Could you check a few things on this model? Use its own coordinates, in mm. Face numbers are marked on the shaded views. A direction names the side the tool comes from. Give positions to 0.01 mm unless a question says otherwise; leave off trailing zeros. Write each loop counter-clockwise with the first axis right and the second up, starting at its lowest first coordinate (ties: lowest second). Pieces come first, ordered by that corner, then holes. Notation, with made-up numbers: M -1.5,-16.5 L 51.5,-16.5 A21 ccw 51.5,13.5 Z; hole C -36.5,56 d7. An arc over 180 degrees is marked long. One line per item, written item: value.
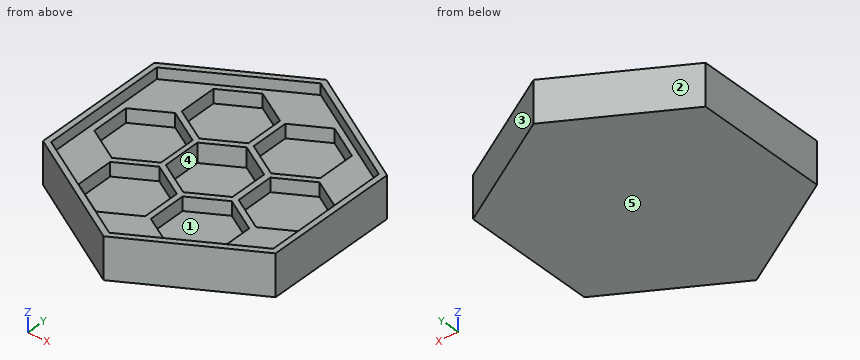
```python
from build123d import *

# Parameters (mm, degrees)
F1_DEPTH = 15
F2_DEPTH = 11
F3_DEPTH = 4
F4_DEPTH = 2


with BuildPart() as f1:
    # F0 (on Top) → F1 (new body)
    with BuildSketch(Plane.XY):
        Polygon((42.0776976909, 24.1136342559), (0.1558290023, 48.4971722611), (-41.9218686887, 24.3835380051), (-42.0776976909, -24.1136342559), (-0.1558290023, -48.4971722611), (41.9218686887, -24.3835380051), align=None)
        Polygon((-40, 23.0940107676), (0, 46.1880215352), (40, 23.0940107676), (40, -23.0940107676), (0, -46.1880215352), (-40, -23.0940107676), align=None, mode=Mode.SUBTRACT)
    extrude(amount=F1_DEPTH)

    # F0 (on Top) → F2 (join)
    with BuildSketch(Plane.XY):
        Polygon((40, 23.0940107676), (0, 46.1880215352), (-40, 23.0940107676), (-40, -23.0940107676), (0, -46.1880215352), (40, -23.0940107676), align=None)
        Polygon((-12.8555934585, -8.7122082831), (-0.8555934585, -15.6404115134), (-0.8555934585, -29.4968179739), (-12.8555934585, -36.4250212042), (-24.8555934585, -29.4968179739), (-24.8555934585, -15.6404115134), align=None, mode=Mode.SUBTRACT)
        Polygon((13.1444065415, -8.6082997926), (25.1444065415, -15.5365030229), (25.1444065415, -29.3929094834), (13.1444065415, -36.3211127137), (1.1444065415, -29.3929094834), (1.1444065415, -15.5365030229), align=None, mode=Mode.SUBTRACT)
        Polygon((-25.7656060661, 13.8564064606), (-13.7656060661, 6.9282032303), (-13.7656060661, -6.9282032303), (-25.7656060661, -13.8564064606), (-37.7656060661, -6.9282032303), (-37.7656060661, 6.9282032303), align=None, mode=Mode.SUBTRACT)
        Polygon((-12.882803033, 36.4407306594), (-0.882803033, 29.5125274291), (-0.882803033, 15.6561209685), (-12.882803033, 8.7279177383), (-24.882803033, 15.6561209685), (-24.882803033, 29.5125274291), align=None, mode=Mode.SUBTRACT)
        Polygon((0, 13.8564064606), (12, 6.9282032303), (12, -6.9282032303), (0, -13.8564064606), (-12, -6.9282032303), (-12, 6.9282032303), align=None, mode=Mode.SUBTRACT)
        Polygon((13.117196967, 36.3054032585), (25.117196967, 29.3772000282), (25.117196967, 15.5207935677), (13.117196967, 8.5925903374), (1.117196967, 15.5207935677), (1.117196967, 29.3772000282), align=None, mode=Mode.SUBTRACT)
        Polygon((26.2343939339, 13.8564064606), (38.2343939339, 6.9282032303), (38.2343939339, -6.9282032303), (26.2343939339, -13.8564064606), (14.2343939339, -6.9282032303), (14.2343939339, 6.9282032303), align=None, mode=Mode.SUBTRACT)
    extrude(amount=F2_DEPTH)

    # F0 (on Top) → F3 (join)
    with BuildSketch(Plane.XY):
        Polygon((25.117196967, 15.5207935677), (25.117196967, 29.3772000282), (13.117196967, 36.3054032585), (1.117196967, 29.3772000282), (1.117196967, 15.5207935677), (13.117196967, 8.5925903374), align=None)
        Polygon((-0.882803033, 15.6561209685), (-0.882803033, 29.5125274291), (-12.882803033, 36.4407306594), (-24.882803033, 29.5125274291), (-24.882803033, 15.6561209685), (-12.882803033, 8.7279177383), align=None)
        Polygon((-13.7656060661, -6.9282032303), (-13.7656060661, 6.9282032303), (-25.7656060661, 13.8564064606), (-37.7656060661, 6.9282032303), (-37.7656060661, -6.9282032303), (-25.7656060661, -13.8564064606), align=None)
        Polygon((12, -6.9282032303), (12, 6.9282032303), (0, 13.8564064606), (-12, 6.9282032303), (-12, -6.9282032303), (0, -13.8564064606), align=None)
        Polygon((38.2343939339, -6.9282032303), (38.2343939339, 6.9282032303), (26.2343939339, 13.8564064606), (14.2343939339, 6.9282032303), (14.2343939339, -6.9282032303), (26.2343939339, -13.8564064606), align=None)
        Polygon((25.1444065415, -29.3929094834), (25.1444065415, -15.5365030229), (13.1444065415, -8.6082997926), (1.1444065415, -15.5365030229), (1.1444065415, -29.3929094834), (13.1444065415, -36.3211127137), align=None)
        Polygon((-0.8555934585, -29.4968179739), (-0.8555934585, -15.6404115134), (-12.8555934585, -8.7122082831), (-24.8555934585, -15.6404115134), (-24.8555934585, -29.4968179739), (-12.8555934585, -36.4250212042), align=None)
    extrude(amount=F3_DEPTH)

    # F4 (add): faces of the model
    f4_faces = [f1.faces().sort_by_distance(p)[0] for p in [
        (-25.7656060661, 0, 4),
        (-12.882803033, 22.5843241988, 4),
        (13.117196967, 22.448996798, 4),
        (26.2343939339, 0, 4),
        (13.1444065415, -22.4647062531, 4),
        (-12.8555934585, -22.5686147437, 4),
    ]]
    extrude(f4_faces, amount=F4_DEPTH)


solid = f1.part
```
1) If we section it at B-B, the plane y = -31: Write out the boundary of the cut face in (x, z), then the cut area to 3 significant figures.
Outcome:
outline: M -30.24,0 L 30.38,0 L 30.38,15 L 26.31,15 L 26.31,11 L 22.36,11 L 22.36,6 L 3.93,6 L 3.93,11 L -3.46,11 L -3.46,6 L -22.25,6 L -22.25,11 L -26.31,11 L -26.31,15 L -30.24,15 Z
area: 513 mm^2
2) On a 3-axis mill with a long thin cutter (end or side, diameter ignored), from which of +Z, -Z, +X, -X, +Y, -Y can I reach the whole of each face in a straight line? I mean the marked faces 1 and 2. Say none if no direction works.
Outcome:
face 1: +Z
face 2: +Z, -Z, -X, +Y
3) We'd pull the mould along X, two halves only. Please class the marked faces 3, 4 and 5: pulls with the +X half, pulls with the -X half, needs draft (parallel to the pull), parting line crosses it, or undercut.
Outcome:
face 3: pulls with the +X half
face 4: undercut
face 5: needs draft
4) If we section it at D-D, the plane z = 8.5: Give the number of separate pieces and of enclosed holes in the cut face, then the cut area to 3 significant figures.
Outcome:
separate pieces: 1
enclosed holes: 7
area: 2,620 mm^2
5) If we section it at A-A, the plane z = 1.25: Write out the boundary of the cut face in (x, y), then the cut area to 3 significant figures.
Outcome:
outline: M -42.08,-24.11 L -0.16,-48.5 L 41.92,-24.38 L 42.08,24.11 L 0.16,48.5 L -41.92,24.38 Z
area: 6,110 mm^2
6) If we section it at C-C, the plane x = 10.5: Write out the boundary of the cut face in (y, z), then the cut area to 3 significant figures.
Outcome:
outline: M -42.39,0 L 42.48,0 L 42.48,15 L 40.13,15 L 40.13,11 L 34.79,11 L 34.79,6 L 10.1,6 L 10.1,11 L 7.79,11 L 7.79,4 L -7.79,4 L -7.79,11 L -10.14,11 L -10.14,6 L -34.79,6 L -34.79,11 L -40.13,11 L -40.13,15 L -42.39,15 Z
area: 596 mm^2
7) Please list where these lines run through material, in increasing order: L1, parallel to X at y = -22, z = 6.75; L2, parallel to X at y = -0.5, z = 9.5; L3, parallel to Y at x = 15, z = 8. Write a range as from..to.
Outcome:
L1: x = -42.07..-24.86, -0.86..1.14, 25.14..41.93
L2: x = -42..-37.77, -13.77..-12, 12..14.23, 38.23..42
L3: y = -39.81..-35.25, -9.68..-7.37, 7.37..9.68, 35.22..39.86
8) I'm going to push flat-ended pins straight in: pin 1 (8 mm diameter, centred on x = -1, y = -25.5, fed in from -Z); pin 2 (2.5 mm diameter, centred on y = 20, z = 7.5, fed in from +X); pin 3 (2.5 mm diameter, centred on y = 1.5, z = 7.5, fed in from +X); pin 4 (12 mm diameter, centred on x = -4, y = 19, fed in from +Z). Where does each tip first touch, or does it pass through?
Outcome:
pin 1: stops at z = 0
pin 2: stops at x = 42.07
pin 3: stops at x = 42.01
pin 4: stops at z = 11
